Geometry check sheet. Reference: the model listing, model coordinates, mm. Round coordinates to 2 decimals unless told otherwise and drop trailing zeros.
from build123d import *

# Parameters (mm, degrees)
SKETCH1_W           = 30
SKETCH1_H           = 30
BOSS_EXTRUDE1_DEPTH = 950
SKETCH2_R           = 2.5
CUT_EXTRUDE1_DEPTH  = 30
SKETCH4_W           = 25
SKETCH4_H           = 25
CUT_EXTRUDE3_DEPTH  = 12


with BuildPart() as part:
    # Sketch1 → Boss-Extrude1 (new body)
    with BuildSketch(Plane.XY):
        Rectangle(SKETCH1_W, SKETCH1_H)
    extrude(amount=BOSS_EXTRUDE1_DEPTH)

    # Sketch2 → Cut-Extrude1 (cut)
    with BuildSketch(Plane(origin=(0, 15, 0), x_dir=(1, 0, 0), z_dir=(0, 1, 0))):
        with Locations(Location((-10, -925, 0), (0, 0, 270))):
            Circle(SKETCH2_R)
        with Locations(Location((10, -925, 0), (0, 0, 270))):
            Circle(SKETCH2_R)
        with Locations(Location((10, -945, 0), (0, 0, 270))):
            Circle(SKETCH2_R)
        with Locations(Location((-10, -945, 0), (0, 0, 270))):
            Circle(SKETCH2_R)
        with Locations(Location((-10, -5, 0), (0, 0, 270))):
            Circle(SKETCH2_R)
        with Locations(Location((10, -5, 0), (0, 0, 270))):
            Circle(SKETCH2_R)
        with Locations(Location((10, -25, 0), (0, 0, 270))):
            Circle(SKETCH2_R)
        with Locations(Location((-10, -25, 0), (0, 0, 270))):
            Circle(SKETCH2_R)
    extrude(amount=-CUT_EXTRUDE1_DEPTH, mode=Mode.SUBTRACT)

    # Sketch4 → Cut-Extrude3 (cut)
    with BuildSketch(Plane(origin=(15, 0, 0), x_dir=(0, 0, -1), z_dir=(1, 0, 0))):
        with Locations((-112.5, 0)):
            Rectangle(SKETCH4_W, SKETCH4_H)
    extrude(amount=-CUT_EXTRUDE3_DEPTH, mode=Mode.SUBTRACT)


solid = part.part
1. Release check for a two-part mould opening along Y. For faces 1 (the face through (0, -15, 468)), 2 (the face through (3, 0, 113)), 3 (the face through (0, 0, 950)) record: +Y half, -Y half, draft (parallel to the pull), parting line (faces both ways), or undercut.
2. Section check A-A (y = -1.75). State how many separate pieces and enclosed holes the cut face has, plus the area to 3 significant figures.
3. Depth check by flat-ended pin: pin 1 Ø8 at (x, z) = (-10, 5) entering from +Y. Enter the tip coordinate at first touch or a pass-through.
4. Scan lines: line 1 along X through (y, z) = (0.75, 25); line 2 along Z through (x, y) = (-10.75, -9.25); line 3 along Z through (x, y) = (-11.5, -11.5). Record each from-to range of solid material in increasing order.
Results below:
1. face 1: -Y half
1. face 2: undercut
1. face 3: draft
2. separate pieces: 1
2. enclosed holes: 8
2. area: 28,000 mm2
3. pin 1: stops at y = 15
4. line 1: x = -15 to -12.5, -7.5 to 7.5, 12.5 to 15
4. line 2: z = 0 to 2.62, 7.38 to 22.62, 27.38 to 922.62, 927.38 to 942.62, 947.38 to 950
4. line 3: z = 0 to 3, 7 to 23, 27 to 923, 927 to 943, 947 to 950
